from build123d import *

# Parameters (mm, degrees)
SKETCH1_R           = 2.286
SKETCH1_W           = 12.7
SKETCH1_H           = 3.81
BOSS_EXTRUDE1_DEPTH = 3.175
FILLET1_R           = 2.54


with BuildPart() as part:
    # Sketch1 → Boss-Extrude1 (new, symmetric)
    with BuildSketch(Plane.XY):
        Polygon((-2.54, -4.445), (2.54, -4.445), (2.54, -6.985), (15.24, -19.05), (25.4, -19.05), (25.4, 19.05), (15.24, 19.05), (2.54, 6.985), (2.54, 4.445), (-2.54, 4.445), (-2.54, 6.985), (-15.24, 19.05), (-25.4, 19.05), (-25.4, -19.05), (-15.24, -19.05), (-2.54, -6.985), align=None)
        with Locations((-20.32, -12.7)):
            Circle(SKETCH1_R, mode=Mode.SUBTRACT)
        with Locations(Location((-20.32, 12.7, 0), (0, 0, 180))):
            Circle(SKETCH1_R, mode=Mode.SUBTRACT)
        with Locations((20.32, 12.7)):
            Circle(SKETCH1_R, mode=Mode.SUBTRACT)
        with Locations(Location((20.32, -12.7, 0), (0, 0, 180))):
            Circle(SKETCH1_R, mode=Mode.SUBTRACT)
        with Locations((-11.43, 3.81)):
            Rectangle(SKETCH1_W, SKETCH1_H, mode=Mode.SUBTRACT)
        with Locations((-11.43, -3.81)):
            Rectangle(SKETCH1_W, SKETCH1_H, mode=Mode.SUBTRACT)
        with Locations((11.43, -3.81)):
            Rectangle(SKETCH1_W, SKETCH1_H, mode=Mode.SUBTRACT)
        with Locations((11.43, 3.81)):
            Rectangle(SKETCH1_W, SKETCH1_H, mode=Mode.SUBTRACT)
    extrude(amount=BOSS_EXTRUDE1_DEPTH, both=True)

    # Fillet1
    fillet1_edges = [part.edges().sort_by_distance(p)[0] for p in [
        (-2.54, -6.985, 0),
        (-15.24, -19.05, 0),
        (-25.4, -19.05, 0),
        (-25.4, 19.05, 0),
        (-15.24, 19.05, 0),
        (-2.54, 6.985, 0),
        (2.54, 6.985, 0),
        (15.24, 19.05, 0),
        (25.4, 19.05, 0),
        (25.4, -19.05, 0),
        (15.24, -19.05, 0),
        (2.54, -6.985, 0),
    ]]
    fillet(fillet1_edges, radius=FILLET1_R)


solid = part.part
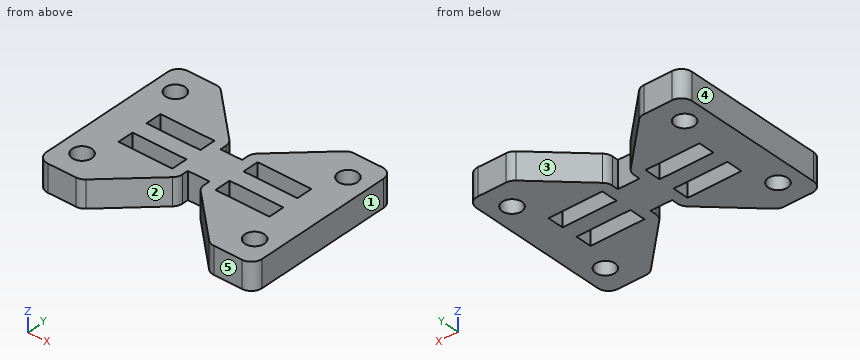
Source: CAD feature listing. Evaluate the final solid. Frame: model axes, mm. Face numbers are marked on the shaded views. A direction names the side the tool comes from. Coordinates: 2 decimals unless noted, no trailing zeros. Loops run counter-clockwise (first coordinate to the right, second up) from the corner with the lowest first, then second, coordinate; pieces in that order, holes last. Notation, with made-up numbers: M -19,63.25 L 9,63.25 A18 cw 9,69.25 Z; hole C 39.5,-13.5 d10. An arc over 180 degrees is marked long. Answer in a Markdown table with one row per item.
Q1. Section B-B on y = -12.7. Return the cut outline in (x, z) (3 decimals), plus the area to 3 significant figures.
Answers below:
| item | result |
|---|---|
| outline | M -25.4,-3.175 L -22.606,-3.175 L -22.606,3.175 L -25.4,3.175 Z; M -18.034,-3.175 L -8.556,-3.175 L -8.556,3.175 L -18.034,3.175 Z; M 8.556,-3.175 L 18.034,-3.175 L 18.034,3.175 L 8.556,3.175 Z; M 22.606,-3.175 L 25.4,-3.175 L 25.4,3.175 L 22.606,3.175 Z |
| area | 156 mm^2 |
Q2. Section D-D on z = -0.75. State how many separate pieces and enclosed holes the cut face has, plus the area to 3 significant figures.
Answers below:
| item | result |
|---|---|
| separate pieces | 1 |
| enclosed holes | 8 |
| area | 1,210 mm^2 |
Q3. Set-up query: the marked faces 1 and 2. Return all of +Z, -Z, +X, -X, +Y, -Y with unobstructed straight access to the full face (end or side cutting, diameter ignored); none if empty.
Answers below:
| item | result |
|---|---|
| face 1 | +Z, -Z, +X, +Y, -Y |
| face 2 | +Z, -Z, -Y |
Q4. Ray query, probe 1 along Y at (x, z) = (-20.32, -0.5); probe 2 along Y at (x, z) = (17, 0) (3 decimals); probe 3 along X at (y, z) = (2, -0.5). Return the intervals inside material, ascending. Write a range as from..to.
Answers below:
| item | result |
|---|---|
| probe 1 | y = -19.05..-14.99, -10.41..10.41, 14.99..19.05 |
| probe 2 | y = -19.05..-5.715, -1.905..1.905, 5.715..19.05 |
| probe 3 | x = -25.4..-17.78, -5.08..5.08, 17.78..25.4 |
Q5. First-contact query: pin 1 (8 mm diameter, centred on x = 9.5, y = -5.5, fed in from +Z) (3 decimals); pin 2 (4 mm diameter, centred on x = 20.32, y = 12.7, fed in from +Z); pin 3 (1.5 mm diameter, centred on x = -8.5, z = 1.5, fed in from -Y); pin 4 (1.9 mm diameter, centred on x = -11, z = 0.5, fed in from +Y). Flat tips, straight axial feed; report the tip coordinate or a pass-through.
Answers below:
| item | result |
|---|---|
| pin 1 | stops at z = 3.175 |
| pin 2 | passes through |
| pin 3 | stops at y = -13.36 |
| pin 4 | stops at y = 15.92 |
Q6. Section A-A on x = 20.32. Return the cut outline in (y, z) (3 decimals).
Answers below:
| item | result |
|---|---|
| outline | M -19.05,-3.175 L -14.986,-3.175 L -14.986,3.175 L -19.05,3.175 Z; M -10.414,-3.175 L 10.414,-3.175 L 10.414,3.175 L -10.414,3.175 Z; M 14.986,-3.175 L 19.05,-3.175 L 19.05,3.175 L 14.986,3.175 Z |
Q7. Section C-C on x = -22. Return the cut outline in (y, z) (3 decimals).
Answers below:
| item | result |
|---|---|
| outline | M -19.05,-3.175 L -14.25,-3.175 L -14.25,3.175 L -19.05,3.175 Z; M -11.15,-3.175 L 11.15,-3.175 L 11.15,3.175 L -11.15,3.175 Z; M 14.25,-3.175 L 19.05,-3.175 L 19.05,3.175 L 14.25,3.175 Z |
Q8. Draft query along X for the marked faces 3, 4 and 5. Return one class per face: pulls with the +X half, pulls with the -X half, needs draft (parallel to the pull), parting line crosses it, or undercut.
Answers below:
| item | result |
|---|---|
| face 3 | undercut |
| face 4 | pulls with the -X half |
| face 5 | needs draft |
